Could you check a few things on this model? Use its own coordinates, in mm. A direction names the side the tool comes from. Coordinates: 2 decimals unless noted, no trailing zeros. Loops run counter-clockwise (first coordinate to the right, second up) from the corner with the lowest first, then second, coordinate; pieces in that order, holes last. Notation, with made-up numbers: (60, -9.5) -> (105, -9.5) arc R24 ccw to (105, 16.5) -> close; hole circle Ø10 at (24, 49). An arc over 180 degrees is marked (long way). One line per question, with ' | ' between items.
Autodesk Inventor part; units mm, degrees
ref_plane "YZ Plane" through (0, 0, 0) normal (1, 0, 0) x (0, 1, 0)
ref_plane "XZ Plane" through (0, 0, 0) normal (0, 1, 0) x (-1, 0, 0)
ref_plane "XY Plane" through (0, 0, 0) normal (0, 0, 1) x (1, 0, 0)
sketch "Sketch1" plane through (0, 0, 0) normal (0, 0, 1) x (1, 0, 0)
  line L0 (-15.7, 12.7) -> (-12.7, 12.7)
  line L1 (-12.7, 12.7) -> (-12.7, -9.7)
  line L2 (-12.7, -9.7) -> (12.7, -9.7)
  line L3 (12.7, -9.7) -> (12.7, 12.7)
  line L4 (12.7, 12.7) -> (15.7, 12.7)
  line L5 (15.7, 12.7) -> (15.7, -12.7)
  line L6 (15.7, -12.7) -> (-15.7, -12.7)
  line L7 (-15.7, -12.7) -> (-15.7, 12.7)
  point P0 (0, 0)
  dimension "d0" = 3
  dimension "d2" = 3
  dimension "d3" = 25.4
  dimension "d4" = 31.4
  dimension "d5" = 15.7
  dimension "d7" = 12.7
  dimension "d8" = 3
extrude "Extrusion1" add sketch "Sketch1" against normal blind 457.2
sketch "Sketch6" plane through (-15.7, -12.7, 0) normal (0, -1, 0) x (1, 0, 0)
  circle A0 centre (16.6513, -447.9) radius 3.175
  point P0 (15.7, 0)
  dimension "d21" = 6.35
extrude "Extrusion4" cut sketch "Sketch6" against normal blind 10
sketch "Sketch7" plane through (-15.7, -12.7, 0) normal (0, -1, 0) x (1, 0, 0)
  line L0 (31.4, -134) -> (0, -134) construction
  line L1 (31.4, -184) -> (0, -184) construction
  line L2 (0, -184) -> (0, -134) construction
  line L3 (0, -159) -> (15.7, -159) construction
  line L4 (15.7, -159) -> (15.7, -184) construction
  circle A0 centre (15.7, -159) radius 3.175
  point P0 (15.7, 0)
  dimension "d25" = 6.35
extrude "Extrusion5" cut sketch "Sketch7" against normal blind 10
sketch "Sketch8" plane through (-15.7, -12.7, 0) normal (0, -1, 0) x (1, 0, 0)
  circle A0 centre (16.6513, -9.3) radius 3.175
  circle A1 centre (15.7, -29) radius 3.175
  circle A2 centre (16.6513, -9.3) radius 3.175
  circle A3 centre (15.7, -29) radius 3.175
  circle A4 centre (15.7, -159) radius 3.175
  circle A5 centre (16.6513, -447.9) radius 3.175
  line L0 (31.4, 0) -> (0, 0)
  line L1 (0, 0) -> (0, -457.2)
  line L2 (31.4, -457.2) -> (0, -457.2)
  line L3 (31.4, 0) -> (31.4, -457.2)
  circle A6 centre (15.7, -268.2855) radius 12.1666
  point P0 (15.7, 0)
  point P1 (15.7, 0)
  dimension "d33" = 188.9145
  dimension "d34" = 15.7
  dimension "d35" = 31.4
extrude "Extrusion6" cut sketch "Sketch8" against normal blind 10 contours A0 | A1 | A6
equation "\"d2\" = d0"
equation "\"d8\" = d0"
equation "\"d34\" = 0.5 * d35"
properties part number "18in C-Channel Rear" material "Aluminum 6061"
Q1. Please list where these lines run through material, in increasing order: L1, parallel to X at y = -4.75, z = -109; L2, parallel to Z at x = 0, y = -11.5 (3 decimals); L3, parallel to X at y = -10.7, z = -159 (3 decimals). Write a range as [from, to].
Values follow:
L1: x = [-15.7, -12.7], [12.7, 15.7] | L2: z = [-457.2, -450.929], [-444.871, -280.452], [-256.119, -162.175], [-155.825, -32.175], [-25.825, -12.329], [-6.271, 0] | L3: x = [-15.7, -3.175], [3.175, 15.7]
Q2. Imagine slicing it at B-B on z = -201. Write out the boundary of the cut face in (x, y).
Values follow:
outline: (-15.7, -12.7) -> (15.7, -12.7) -> (15.7, 12.7) -> (12.7, 12.7) -> (12.7, -9.7) -> (-12.7, -9.7) -> (-12.7, 12.7) -> (-15.7, 12.7) -> close
Q3. Imagine slicing it at A-A on y = 3.75. Write out the boundary of the cut face in (x, z), plus the area to 3 significant figures.
Values follow:
outline: (-15.7, -457.2) -> (-12.7, -457.2) -> (-12.7, 0) -> (-15.7, 0) -> close; (12.7, -457.2) -> (15.7, -457.2) -> (15.7, 0) -> (12.7, 0) -> close | area: 2,740 mm2
Q4. We'd pull the mould along X, two halves only. Please class faces 3 (the face through (15.7, 0, -225)), 4 (the face through (0, -12.7, -225)), 5 (the face through (-1.58, -11.22, -256.22)), 6 (the face through (-15.7, 0, -225)): released by +X, released by -X, zero draft, split by the parting line, or undercut.
Values follow:
face 3: released by +X | face 4: zero draft | face 5: undercut | face 6: released by -X
Q5. For faces 1 (the face through (12.7, 1, -225)), 2 (the face through (0, -10, -457.2)), which set-ups out of +Z, -Z, +X, -X, +Y, -Y let a thin tool reach every point of the face, with its end or its side?
Values follow:
face 1: +Z, -Z, +Y | face 2: -Z, +X, -X, +Y, -Y
Q6. For pin 1 (5 mm diameter, centred on x = 0, z = -29, fed in from +Y), with a flat end and sliding along its axis, tell me the tip position at first contact or that it passes through.
Values follow:
pin 1: passes through
